Could you check a few things on this model? Use its own coordinates, in mm. Face numbers are marked on the shaded views. A direction names the side the tool comes from. Coordinates: 2 decimals unless noted, no trailing zeros. Order: outer loops, then holes, each group sorted by start corner. A loop starts at its lowest first (then second) coordinate and runs counter-clockwise, first axis right, second up. Notation, with made-up numbers: (-18, 38.25) -> (30, 38.25) arc R16 ccw to (30, 45.25) -> close; hole circle Ø8 at (35.5, -30.5). An arc over 180 degrees is marked (long way). Put each result on its own line as item: value. Start each with the question number.
Q1. If we section it at C-C (z = -21.5): Please give me the cut outline in (x, y).
Q2. If we section it at B-B (x = -23): Please give me the cut outline in (y, z), and give its area (3 significant figures).
Q3. For the marked faces 1 and 2, which set-ups out of +Z, -Z, +X, -X, +Y, -Y let a thin tool reach every point of the face, with its end or its side?
Q4. Please list where these lines run through material, in increasing order: line 1 along X through (y, z) = (-1, -22); line 2 along Z through (x, y) = (-31.5, -4); line 3 along X through (y, z) = (-1.5, -4).
Q5. Will these pins go through, and if not, where does the flat tip stop? pin 1 (3 mm diameter, centred on y = 1.5, z = -25.5, fed in from +X); pin 2 (8 mm diameter, centred on x = -29, z = -5.5, fed in from -Y); pin 3 (3 mm diameter, centred on x = 3.5, y = 2.5, fed in from -Z).
Q6. If we section it at A-A (y = 1): Please give me the cut outline in (x, z) (1 decimal), and give its area (3 significant figures).
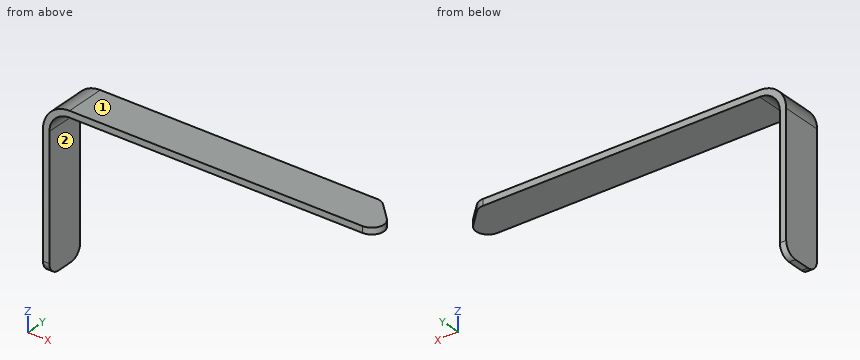
from build123d import *

# Parameters (mm, degrees)
SKETCH1_W                    = 85
SKETCH1_H                    = 10
BOSS_EXTRUDE1_DEPTH          = 1.6
CUT_EXTRUDE1_DEPTH           = 43.823007835
CUT_EXTRUDE1_DEPTH_BACK      = 10
CONVERT_SOLID1_DEPTH         = 0.0125
EDGE_FLANGE1_STRIP_W         = 16.35
EDGE_FLANGE1_STRIP_H         = 1.5875
EDGE_FLANGE1_STRIP_CUT_DEPTH = 10
EDGE_FLANGE1_DEPTH           = 10
FILLET2_R                    = 3


# Read off the part's stored shape, not the designer's step: Convert-Solid1
# Sheet-metal steps are written as plain solids
with BuildPart() as part:
    # Sketch1 → Boss-Extrude1 (new body)
    with BuildSketch(Plane.XY):
        Rectangle(SKETCH1_W, SKETCH1_H)
    extrude(amount=BOSS_EXTRUDE1_DEPTH)

    # Sketch2 → Cut-Extrude1 (cut, two sides: drawn at the far end of the back side and taken through both)
    with BuildSketch(Plane.XY.offset(1.6).offset(-CUT_EXTRUDE1_DEPTH_BACK)):
        Polygon((32.5, 5), (42.5, -5), (42.5, 5), align=None)
    extrude(amount=CUT_EXTRUDE1_DEPTH + CUT_EXTRUDE1_DEPTH_BACK, mode=Mode.SUBTRACT)

    # Convert-Solid1 outline → Convert-Solid1 (cut)
    with BuildSketch(Plane.XY):
        Polygon((32.5, 5), (-42.5, 5), (-42.5, -5), (42.5, -5), align=None)
    extrude(amount=CONVERT_SOLID1_DEPTH, mode=Mode.SUBTRACT)

    # Edge-Flange1 strip (across the edge) → Edge-Flange1 strip cut (cut)
    with BuildSketch(Plane(origin=(-42.5, -5, 0.0125), x_dir=(1, 0, 0), z_dir=(0, 1, 0))):
        with Locations((-3.175, -0.79375)):
            Rectangle(EDGE_FLANGE1_STRIP_W, EDGE_FLANGE1_STRIP_H)
    extrude(amount=EDGE_FLANGE1_STRIP_CUT_DEPTH, mode=Mode.SUBTRACT)

    # Edge-Flange1 section (across the edge) → Edge-Flange1 (add)
    with BuildSketch(Plane(origin=(-42.5, -5, 0.0125), x_dir=(1, 0, 0), z_dir=(0, 1, 0))):
        with BuildLine():
            Line((-1.5875, 5), (-1.5875, 38.4125))
            Line((-1.5875, 38.4125), (0, 38.4125))
            Line((0, 38.4125), (0, 5))
            ThreePointArc((0, 5), (1.464466094, 1.464466094), (5, 0))
            Line((5, 0), (5, -1.5875))
            ThreePointArc((5, -1.5875), (0.341934079, 0.341934079), (-1.5875, 5))
        make_face()
    extrude(amount=EDGE_FLANGE1_DEPTH)

    # Fillet2
    fillet2_edges = [part.edges().sort_by_distance(p)[0] for p in [
        (-43.29375, -5, -38.4),
        (-43.29375, 5, -38.4),
        (42.5, -5, 0.80625),
        (32.5, 5, 0.80625),
    ]]
    fillet(fillet2_edges, radius=FILLET2_R)


solid = part.part
The answers:
1. outline: (-44.09, -5) -> (-42.5, -5) -> (-42.5, 5) -> (-44.09, 5) -> close
2. outline: (-5, 0.01) -> (5, 0.01) -> (5, 1.6) -> (-5, 1.6) -> close
2. area: 15.9 mm^2
3. face 1: +Z, +X, -X, +Y, -Y
3. face 2: -Z, +X, +Y, -Y
4. line 1: -44.09 to -42.5
4. line 2: 0.01 to 1.6
4. line 3: -44.01 to -42.4
5. pin 1: x = -42.5
5. pin 2: through
5. pin 3: z = 0.01
6. outline: (-44.1, -38.4) -> (-42.5, -38.4) -> (-42.5, -5) arc R5 cw to (-37.5, 0) -> (36.5, 0) -> (36.5, 1.6) -> (-37.5, 1.6) arc R6.6 ccw to (-44.1, -5) -> close
6. area: 185 mm^2
